from build123d import *

# Parameters (mm, degrees)
EXTRUDE_1_DEPTH           = 14.5
EXTRUDE_2_REACH           = 54.409
CUT_EXTRUDE_2_DEPTH       = 6.5
CUT_EXTRUDE_4_DEPTH       = 1.2
CUT_EXTRUDE_5_DEPTH       = 6.45
CUT_EXTRUDE_6_REACH       = 46.446
SKETCH_12_R               = 1.45
CUT_EXTRUDE_START         = -11.3
CUT_EXTRUDE_9_DEPTH       = 11.3
CUT_EXTRUDE_10_DEPTH      = 10
CUT_EXTRUDE_10_DEPTH_BACK = 45.446455555
SKETCH_17_R               = 1.45
EXTRUDE_START             = 1
SKETCH_18_R               = 1.2
EXTRUDE_3_DEPTH           = 1
CUT_EXTRUDE_11_REACH      = 54.409
SKETCH_20_R               = 1.2
EXTRUDE_4_DEPTH           = 4.5
SKETCH_23_W               = 4
SKETCH_23_H               = 12
CUT_EXTRUDE_13_DEPTH      = 15
CUT_EXTRUDE_14_REACH      = 53.391
SKETCH_24_R               = 2


with BuildPart() as part:
    # 草圖2 → 填料-伸長1 (new body)
    with BuildSketch(Plane.XY.offset(-1.2)):
        with BuildLine():
            Line((3.005790246, 9.65), (27.71, 9.65))
            Line((27.71, 9.65), (27.71, -9.635))
            ThreePointArc((27.71, -9.635), (26.099087297, -13.524087297), (22.21, -15.135))
            Line((22.21, -15.135), (20.682621431, -15.135))
            Line((20.682621431, -15.135), (13.950432746, -23.093384504))
            Line((13.950432746, -23.093384504), (8.257610616, -29.823093007))
            Line((8.257610616, -29.823093007), (-8.232750503, -29.852481121))
            Line((-8.232750503, -29.852481121), (-13.949609825, -23.094357311))
            Line((-13.949609825, -23.094357311), (-19.48563893, -16.55))
            Line((-19.48563893, -16.55), (3.005790246, -16.55))
            Line((3.005790246, -16.55), (7.547371488, -16.55))
            Line((7.547371488, -16.55), (7.547371488, -9.65))
            Line((7.547371488, -9.65), (0.65, -9.65))
            Line((0.65, -9.65), (0.65, 8.289548141))
            ThreePointArc((0.65, 8.289548141), (1.950360965, 8.757709354), (3.005790246, 9.65))
        make_face()
    extrude(amount=EXTRUDE_1_DEPTH)

    # 草圖6 → 填料-伸長2 (add, up to next)
    with BuildSketch(Plane(origin=(0.058521361, -32.837709687, 0), x_dir=(-0.9999984119942069, -0.0017821360960036876, 0), z_dir=(0.0017821360960036876, -0.9999984119942069, 0)), mode=Mode.PRIVATE) as extrude_2_sk1:
        with BuildLine():
            Line((6.040744961, 1.2), (13.990744961, 1.2))
            ThreePointArc((13.990744961, 1.2), (0.040744961, -12.75), (-13.909255039, 1.2))
            Line((-13.909255039, 1.2), (-5.959255039, 1.2))
            ThreePointArc((-5.959255039, 1.2), (0.040744961, -4.8), (6.040744961, 1.2))
        make_face()
    extrude_2_tool1 = extrude(extrude_2_sk1.sketch, amount=-EXTRUDE_2_REACH, mode=Mode.PRIVATE) - part.part
    add(extrude_2_tool1.solids().sort_by_distance((0.017776, -32.837782, 5.486422))[0])

    # 草圖8 → 除料-伸長2 (cut)
    with BuildSketch(Plane(origin=(0.053174952, -29.837714451, 0), x_dir=(0.9999984119942069, 0.0017821360960043932, 0), z_dir=(0.0017821360960043932, -0.9999984119942069, 0))):
        with BuildLine():
            Line((5.959255039, -1.2), (-6.040744961, -1.2))
            ThreePointArc((-6.040744961, -1.2), (-0.040744961, 4.8), (5.959255039, -1.2))
        make_face()
    extrude(amount=-CUT_EXTRUDE_2_DEPTH, mode=Mode.SUBTRACT)

    # 草圖10 → 除料-伸長4 (cut)
    with BuildSketch(Plane(origin=(0, 0, -1.2), x_dir=(-1, 0, 0), z_dir=(0, 0, -1))):
        with BuildLine():
            Line((15.425245412, -16.55), (16.080147592, -16.55))
            Line((16.080147592, -16.55), (8.049473708, -26.043374829))
            ThreePointArc((8.049473708, -26.043374829), (6.88166706, -26.933100433), (5.447606932, -27.24751348))
            Line((5.447606932, -27.24751348), (-5.476193678, -27.228045749))
            ThreePointArc((-5.476193678, -27.228045749), (-6.90363194, -26.911082911), (-8.065941929, -26.023907099))
            Line((-8.065941929, -26.023907099), (-18.792755233, -13.343320029))
            ThreePointArc((-18.792755233, -13.343320029), (-19.478083321, -12.820701245), (-20.319700829, -12.635))
            Line((-20.319700829, -12.635), (-22.21, -12.635))
            ThreePointArc((-22.21, -12.635), (-24.331320344, -11.756320344), (-25.21, -9.635))
            Line((-25.21, -9.635), (-25.21, 9.756016868))
            Line((-25.21, 9.756016868), (-3.090378498, 9.756016868))
            ThreePointArc((-3.090378498, 9.756016868), (-2.008790795, 8.792133036), (-0.65, 8.289548141))
            Line((-0.65, 8.289548141), (-0.65, -9.65))
            Line((-0.65, -9.65), (-7.547371488, -9.65))
            Line((-7.547371488, -9.65), (-7.547371488, -16.55))
            Line((-7.547371488, -16.55), (15.425245412, -16.55))
        make_face()
    extrude(amount=-CUT_EXTRUDE_4_DEPTH, mode=Mode.SUBTRACT)

    # 草圖11 → 除料-伸長5 (cut)
    with BuildSketch(Plane(origin=(0, 0, 2), x_dir=(-1, 0, 0), z_dir=(0, 0, -1))):
        with BuildLine():
            Line((15.425245412, -16.55), (9.998981166, -22.964599963))
            ThreePointArc((9.998981166, -22.964599963), (9.142321056, -23.617873443), (8.090299171, -23.85))
            Line((8.090299171, -23.85), (-8.090299171, -23.85))
            ThreePointArc((-8.090299171, -23.85), (-9.142321056, -23.617873443), (-9.998981166, -22.964599963))
            Line((-9.998981166, -22.964599963), (-15.425245412, -16.55))
            Line((-15.425245412, -16.55), (15.425245412, -16.55))
        make_face()
    extrude(amount=-CUT_EXTRUDE_5_DEPTH, mode=Mode.SUBTRACT)

    # 草圖12 → 除料-伸長6 (cut, up to next)
    with BuildSketch(Plane.XY.offset(2), mode=Mode.PRIVATE) as cut_extrude_6_sk1:
        with Locations((-5.040260671, -20.109460334)):
            Circle(SKETCH_12_R)
    cut_extrude_6_tool1 = extrude(cut_extrude_6_sk1.sketch, amount=-CUT_EXTRUDE_6_REACH, mode=Mode.PRIVATE) & part.part
    # 草圖12 → 除料-伸長6 (cut, up to next)
    with BuildSketch(Plane.XY.offset(2), mode=Mode.PRIVATE) as cut_extrude_6_sk2:
        with Locations((4.959739329, -20.109460334)):
            Circle(SKETCH_12_R)
    cut_extrude_6_tool2 = extrude(cut_extrude_6_sk2.sketch, amount=-CUT_EXTRUDE_6_REACH, mode=Mode.PRIVATE) & part.part
    add(cut_extrude_6_tool1.solids().sort_by_distance((-5.040261, -20.10946, 2))[0], mode=Mode.SUBTRACT)
    add(cut_extrude_6_tool2.solids().sort_by_distance((4.959739, -20.10946, 2))[0], mode=Mode.SUBTRACT)

    # 草圖16 → 除料-伸長9 (cut)
    with BuildSketch(Plane.XY.offset(13.3).offset(CUT_EXTRUDE_START)):
        with BuildLine():
            Line((27.71, 9.65), (17.635, 9.65))
            Line((17.635, 9.65), (17.635, -9.65))
            Line((17.635, -9.65), (7.547371488, -9.65))
            Line((7.547371488, -9.65), (7.547371488, -16.55))
            Line((7.547371488, -16.55), (19.48563893, -16.55))
            Line((19.48563893, -16.55), (20.682621431, -15.135))
            Line((20.682621431, -15.135), (22.21, -15.135))
            ThreePointArc((22.21, -15.135), (26.099087297, -13.524087297), (27.71, -9.635))
            Line((27.71, -9.635), (27.71, 9.65))
        make_face()
    extrude(amount=CUT_EXTRUDE_9_DEPTH, mode=Mode.SUBTRACT)

    # 草圖17 → 除料-伸長10 (cut, two sides: drawn at the far end of the back side and taken through both)
    with BuildSketch(Plane.XY.offset(2).offset(-CUT_EXTRUDE_10_DEPTH_BACK)):
        with Locations(Location((20.81, 5.15, 0), (0, 0, 180))):
            Circle(SKETCH_17_R)
        with Locations(Location((20.81, -5.15, 0), (0, 0, 180))):
            Circle(SKETCH_17_R)
    extrude(amount=CUT_EXTRUDE_10_DEPTH + CUT_EXTRUDE_10_DEPTH_BACK, mode=Mode.SUBTRACT)

    # 草圖18 → 填料-伸長3 (add)
    with BuildSketch(Plane(origin=(0.058521361, -32.837709687, 0), x_dir=(0.9999984119942069, 0.001782136096003688, 0), z_dir=(0.001782136096003688, -0.9999984119942069, 0)).offset(EXTRUDE_START)):
        with BuildLine():
            Line((-1.542184808, 7.30666872), (-2.465462288, 12.537657948))
            ThreePointArc((-2.465462288, 12.537657948), (-0.043106116, 12.7499998), (2.379321799, 12.538477968))
            Line((2.379321799, 12.538477968), (1.457815149, 7.307176495))
            Line((1.457815149, 7.307176495), (-1.542184808, 7.30666872))
        make_face()
        with Locations((-0.042503946, 9.192304697)):
            Circle(SKETCH_18_R, mode=Mode.SUBTRACT)
    extrude(amount=-EXTRUDE_3_DEPTH)

    # 草圖20 → 除料-伸長11 (cut, up to next)
    with BuildSketch(Plane(origin=(0.058521361, -32.837709687, 0), x_dir=(0.9999984119942069, 0.001782136096003688, 0), z_dir=(0.001782136096003688, -0.9999984119942069, 0)), mode=Mode.PRIVATE) as cut_extrude_11_sk1:
        with Locations(Location((-0.042503946, 9.192304697, 0), (0, 0, 218.213041012))):
            Circle(SKETCH_20_R)
    cut_extrude_11_tool1 = extrude(cut_extrude_11_sk1.sketch, amount=-CUT_EXTRUDE_11_REACH, mode=Mode.PRIVATE) & part.part
    add(cut_extrude_11_tool1.solids().sort_by_distance((0.016017, -32.837785, 9.192305))[0], mode=Mode.SUBTRACT)

    # 草圖22 → 填料-伸長4 (add)
    with BuildSketch(Plane.XY.offset(13.3)):
        with BuildLine():
            Line((0.65, 8.289548141), (0.65, -9.65))
            Line((0.65, -9.65), (17.635, -9.65))
            Line((17.635, -9.65), (17.635, 9.65))
            Line((17.635, 9.65), (3.005790246, 9.65))
            ThreePointArc((3.005790246, 9.65), (1.950360965, 8.757709354), (0.65, 8.289548141))
        make_face()
    extrude(amount=EXTRUDE_4_DEPTH)

    # 草圖23 → 除料-伸長13 (cut)
    with BuildSketch(Plane.ZY.offset(-0.65)):
        with Locations((15, 0)):
            Rectangle(SKETCH_23_W, SKETCH_23_H)
    extrude(amount=-CUT_EXTRUDE_13_DEPTH, mode=Mode.SUBTRACT)

    # 除料-伸長14: up to this plane
    cut_extrude_14_end = Plane(origin=(3.005790246, -16.55, 13.3), z_dir=(0, -1, 0))
    # 草圖24 → 除料-伸長14 (cut, up to the surface)
    with BuildSketch(Plane(origin=(0.053174952, -29.837714451, 0), x_dir=(0.9999984119942069, 0.0017821360960043932, 0), z_dir=(0.0017821360960043932, -0.9999984119942069, 0)), mode=Mode.PRIVATE) as cut_extrude_14_sk1:
        with Locations((0, 15.066296733)):
            Circle(SKETCH_24_R)
    cut_extrude_14_tool1 = split(extrude(cut_extrude_14_sk1.sketch, amount=-CUT_EXTRUDE_14_REACH, mode=Mode.PRIVATE), bisect_by=cut_extrude_14_end, keep=Keep.BOTH, mode=Mode.PRIVATE)
    add(cut_extrude_14_tool1.solids().sort_by_distance((0.053175, -29.837714, 15.066297))[0], mode=Mode.SUBTRACT)


solid = part.part
For this review, take the finished solid that the model builds, in its own axes (mm). A direction names the side the tool comes from. Give positions to 0.01 mm unless a question says otherwise; leave off trailing zeros. Write each loop counter-clockwise with the first axis right and the second up, starting at its lowest first coordinate (ties: lowest second). Pieces come first, ordered by that corner, then holes. Notation, with made-up numbers: (65.25, 42) -> (100.25, 42) arc R29 ccw to (100.25, 71) -> close; hole circle Ø3 at (63.5, 53.25). An arc over 180 degrees is marked (long way). Use CSV: the item, a comma, the result in double quotes.
Q1. For P1, Ø1.7, axis at x = -5.04, y = -20.11, coming from the +Z side; P2, Ø8, axis at x = 9, z = 1, coming from the -Y side; P3, Ø1.9, axis at x = -3, z = 5.5, coming from the +Y side, all flat-tipped, find the tip position at first contact; note any pin that passes through.
Conclusion:
P1,"z = 13.3"
P2,"y = -32.83"
P3,"y = -23.85"
Q2. Mouldability with a two-part tool opening along Z and no side actions: class faces 6 (the face through (8, 6, 15)), 7 (the face through (8, -22, 13.3)), 8 (the face through (17.635, 0, 10)) as pulls with the +Z half, pulls with the -Z half, needs draft (parallel to the pull), parting line crosses it, or undercut.
Conclusion:
face 6,"undercut"
face 7,"pulls with the +Z half"
face 8,"needs draft"
Q3. Take a section at D-D, the plane x = 17. Write out the cut boundary in (y, z).
Conclusion:
outline,"(-19.49, -1.2) -> (-15.46, -1.2) -> (-15.46, 0) -> (9.65, 0) -> (9.65, 17.8) -> (-9.65, 17.8) -> (-9.65, 2) -> (-16.55, 2) -> (-16.55, 13.3) -> (-19.49, 13.3) -> close"
Q4. To check wall thickness, follow probe 1 along Y at (x, z) = (20.81, 1.05) (3 decimals); probe 2 along Z at (x, y) = (11, 5); probe 3 along Y at (x, z) = (5, 7.25). State the ranges of each line that lie inside material, in increasing order. Write a range as [from, to].
Conclusion:
probe 1,"[-15.135, -6.6], [-3.7, 3.7], [6.6, 9.65]"
probe 2,"[0, 13], [17, 17.8]"
probe 3,"[-32.83, -23.85], [-9.65, 9.65]"
Q5. Take a section at A-A, the plane y = -5.15. Write out the cut boundary in (x, z) (3 decimals).
Conclusion:
outline,"(0.65, 0) -> (19.36, 0) -> (19.36, 2) -> (17.635, 2) -> (17.635, 17.8) -> (0.65, 17.8) -> (0.65, 17) -> (15.65, 17) -> (15.65, 13) -> (0.65, 13) -> close; (22.26, 0) -> (25.21, 0) -> (25.21, -1.2) -> (27.71, -1.2) -> (27.71, 2) -> (22.26, 2) -> close"
Q6. Tool access review of faces 1 (the face through (21, -12.635, -1)), 2 (the face through (-6.11, -19.13, 1.01)), 3 (the face through (12.674, -19.802, 5.18)), 4 (the face through (8, -6, 15)), 5 (the face through (13.354, -19.772, -0.608)): name each direction out of +Z, -Z, +X, -X, +Y, -Y from which nothing blocks a thin tool from reaching the whole face with its end or side.
Conclusion:
face 1,"-Z, -X, +Y"
face 2,"-Z"
face 3,"none"
face 4,"-X"
face 5,"-Z, +Y"
Q7. Take a section at B-B, the plane y = 3. Write out the cut boundary in (x, z) (3 decimals).
Conclusion:
outline,"(0.65, 0) -> (25.21, 0) -> (25.21, -1.2) -> (27.71, -1.2) -> (27.71, 2) -> (17.635, 2) -> (17.635, 17.8) -> (0.65, 17.8) -> (0.65, 17) -> (15.65, 17) -> (15.65, 13) -> (0.65, 13) -> close"
Q8. Take a section at C-C, the plane z = 12. Write out the cut boundary in (x, y) (3 decimals).
Conclusion:
outline,"(-19.486, -16.55) -> (-8.233, -29.852) -> (-4.5, -29.846) -> (-4.495, -32.846) -> (-2.312, -32.842) -> (-2.31, -33.842) -> (2.345, -33.834) -> (2.343, -32.834) -> (4.53, -32.83) -> (4.525, -29.83) -> (8.258, -29.823) -> (19.486, -16.55) -> close; (0.65, -9.65) -> (17.635, -9.65) -> (17.635, 9.65) -> (3.006, 9.65) arc R3.9 cw to (0.65, 8.29) -> close"
